Check sheet for the modelled part. Datum: model origin and axes. Units: mm. Round coordinates to 2 decimals unless told otherwise and drop trailing zeros. Order: outer loops, then holes, each group sorted by start corner. A loop starts at its lowest first (then second) coordinate and runs counter-clockwise, first axis right, second up. Notation, with made-up numbers: M -1,11 L 19,11 A6 cw 19,17 Z; hole C 23.25,65 d1. An arc over 180 degrees is marked long. One line per item, written item: value. Start each with the question number.
(1) Depth check by flat-ended pin: pin 1 Ø8 at (y, z) = (-20.5, -13.5) entering from +X. Enter the tip coordinate at first touch or a pass-through.
(2) Cross-section at B-B, the plane z = 53.5. Enter the section's corners in (x, y).
(3) Thickness scan on L1, parallel to X at y = -21.75, z = -34.5; L2, parallel to X at y = -6.75, z = -36.5; L3, parallel to Z at x = 105, y = -17. Record the ranges inside material, lowest first.
(4) Cross-section at A-A, the plane y = -19.5. Enter the section's corners in (x, z), and give its area (3 significant figures).
(5) Cross-section at C-C, the plane x = 84.5. Enter the section's corners in (y, z).
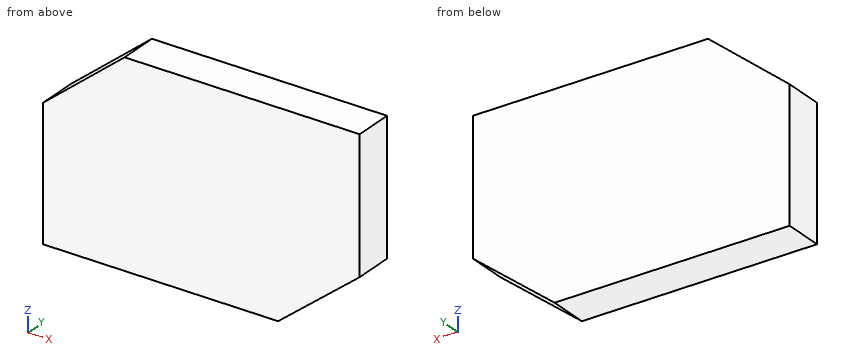
from build123d import *

# Parameters (mm, degrees)
F1_DEPTH = 25.4


with BuildPart() as f1:
    # F0 (on Front) → F1 (new body)
    with BuildSketch(Plane.XZ):
        Polygon((-75.995557, -42.566791), (75.995557, -42.566791), (75.995557, 0), (-18.541871, 0), (-22.720322, 0), align=None)
        Polygon((75.995557, 0), (75.995557, -42.566791), (128.748477, 0), align=None)
        Polygon((-75.995557, 42.566791), (-75.995557, -42.566791), (-22.720322, 0), (-22.978842, 42.566791), align=None)
        Polygon((75.995557, 42.566791), (75.995557, 0), (128.748477, 0), (128.748477, 86.002111), align=None)
        Polygon((-23.242638, 86.002111), (-75.995557, 42.566791), (-22.978842, 42.566791), align=None)
        Polygon((-22.978842, 42.566791), (75.995557, 42.566791), (128.748477, 86.002111), (0, 86.002111), (-23.242638, 86.002111), align=None)
        Polygon((-18.541871, 0), (75.995557, 0), (75.995557, 42.566791), (-22.978842, 42.566791), (-22.720322, 0), align=None)
    extrude(amount=F1_DEPTH)


solid = f1.part
Values found:
1. pin 1: x = 116.98
2. outline: M -62.72,-25.4 L 128.75,-25.4 L 128.75,0 L -62.72,0 Z
3. L1: -76 to 85.99
3. L2: -76 to 83.51
3. L3: -19.16 to 86
4. outline: M -76,-42.57 L 76,-42.57 L 128.75,0 L 128.75,86 L -23.24,86 L -76,42.57 Z
4. area: 24,100 mm^2
5. outline: M -25.4,-35.7 L 0,-35.7 L 0,86 L -25.4,86 Z
